Work out the finished part from the listing and answer in its coordinate system (mm). Coordinates: 2 decimals unless noted, no trailing zeros. Order: outer loops, then holes, each group sorted by start corner. A loop starts at its lowest first (then second) coordinate and runs counter-clockwise, first axis right, second up. Notation, with made-up numbers: M 42,-37.5 L 82,-37.5 A10 ccw 82,-21.5 Z; hole C 9,-1 d9. An arc over 180 degrees is marked long. Answer in a Markdown table with one row per item. Add a question column.
Item 1: Flat-ended cylindrical pins translate along their axes: pin 1 Ø1.6 at (y, z) = (10, 2) entering from -X; pin 2 Ø1.6 at (y, z) = (11.5, 2) entering from +X. Find the tip coordinate at first contact, or state that the pin passes through.
Item 2: Consider line 1 (X direction, y = 24.5, z = 2.7). Determine where the line is inside the solid, lowest interval first. Write a range as from..to.
Item 3: The part is cut by section A-A (z = 0.7). Write down the section's boundary in (x, y) (3 decimals).
Item 4: The part is cut by section B-B (y = 12.5). Write down the section's boundary in (x, z) (3 decimals).
from build123d import *

# Parameters (mm, degrees)
F1_DEPTH = 3.175
F2_DEPTH = 9.525
F3_DEPTH = 9.525


with BuildPart() as f1:
    # F0 (on Top) → F1 (new body)
    with BuildSketch(Plane.XY):
        Polygon((0, 7.62), (0, 0), (101.6, 0), (101.6, 7.62), (88.9, 7.62), (88.9, 15.24), (101.6, 15.24), (101.6, 21.59), (88.9, 21.59), (88.9, 29.21), (101.6, 29.21), (101.6, 35.56), (88.9, 35.56), (88.9, 43.18), (101.6, 43.18), (101.6, 50.8), (0, 50.8), (0, 43.18), (12.7, 43.18), (12.7, 35.56), (0, 35.56), (0, 29.21), (12.7, 29.21), (12.7, 21.59), (0, 21.59), (0, 15.24), (12.7, 15.24), (12.7, 7.62), align=None)
    extrude(amount=F1_DEPTH)

    # F2 (cut): faces of the model
    f2_faces = [f1.faces().sort_by_distance(p)[0] for p in [
        (0, 46.99, 1.5875),
        (0, 32.385, 1.5875),
        (0, 18.415, 1.5875),
        (0, 3.81, 1.5875),
    ]]
    extrude(f2_faces, amount=-F2_DEPTH, mode=Mode.SUBTRACT)

    # F3 (cut): faces of the model
    f3_faces = [f1.faces().sort_by_distance(p)[0] for p in [
        (101.6, 3.81, 1.5875),
        (101.6, 18.415, 1.5875),
        (101.6, 32.385, 1.5875),
        (101.6, 46.99, 1.5875),
    ]]
    extrude(f3_faces, amount=-F3_DEPTH, mode=Mode.SUBTRACT)


solid = f1.part
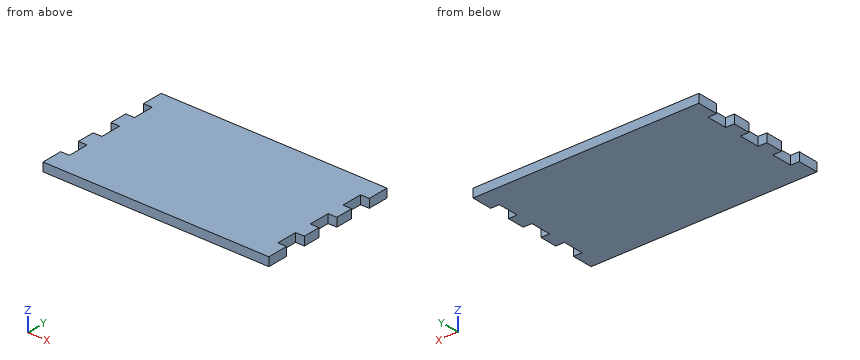
Reply:
| question | item | result |
|---|---|---|
| 1 | pin 1 | stops at x = 12.7 |
| 1 | pin 2 | stops at x = 88.9 |
| 2 | line 1 | x = 12.7..88.9 |
| 3 | outline | M 9.525,0 L 92.075,0 L 92.075,7.62 L 88.9,7.62 L 88.9,15.24 L 92.075,15.24 L 92.075,21.59 L 88.9,21.59 L 88.9,29.21 L 92.075,29.21 L 92.075,35.56 L 88.9,35.56 L 88.9,43.18 L 92.075,43.18 L 92.075,50.8 L 9.525,50.8 L 9.525,43.18 L 12.7,43.18 L 12.7,35.56 L 9.525,35.56 L 9.525,29.21 L 12.7,29.21 L 12.7,21.59 L 9.525,21.59 L 9.525,15.24 L 12.7,15.24 L 12.7,7.62 L 9.525,7.62 Z |
| 4 | outline | M 12.7,0 L 88.9,0 L 88.9,3.175 L 12.7,3.175 Z |
